Source: CAD feature listing. Evaluate the final solid. Frame: model axes, mm. A direction names the side the tool comes from. Round coordinates to 2 decimals unless told otherwise and drop trailing zeros. Write each loop counter-clockwise with the first axis right and the second up, starting at its lowest first coordinate (ties: lowest second). Pieces come first, ordered by that corner, then holes. Notation, with made-up numbers: M -40,22.25 L 2,22.25 A15 cw 2,49.25 Z; hole C -4.5,39 d4. An arc over 180 degrees is marked long. Use a Markdown table: item, result.
```python
from build123d import *

# Parameters (mm, degrees)
F0_W      = 4.724400118
F0_H      = 62.3315982521
F1_DEPTH  = 6.35
F2_R      = 2.53999
F4_DEPTH  = 1.27
F6_DEPTH  = 1.27
F8_DEPTH  = 25.4
F9_DEPTH  = 50.8
F11_DEPTH = 25.4
F13_DEPTH = 25.4
F15_DEPTH = 101.6


# Not quite as in the source:
# - a fillet or chamfer is up to 0.001 mm smaller than in the source, because OpenCascade refuses the exact size


with BuildPart() as f1:
    # F0 (on Top) → F1 (new body)
    with BuildSketch(Plane.XY):
        with Locations((2.362200059, 31.165799126)):
            Rectangle(F0_W, F0_H)
        with Locations((7.086600177, 31.165799126)):
            Rectangle(F0_W, F0_H)
        Polygon((4.724400118, 75.0454813242), (4.724400118, 62.3315982521), (9.448800236, 62.3315982521), align=None)
        Polygon((4.724400118, 75.0454813242), (0, 62.3315982521), (4.724400118, 62.3315982521), align=None)
        with BuildLine():
            Line((4.724400118, 0), (0, 0))
            Line((0, 0), (-20.32, 0))
            ThreePointArc((-20.32, 0), (-18.5239487758, -0.7439487758), (-17.78, -2.54))
            ThreePointArc((-17.78, -2.54), (-18.5239487758, -4.3360512242), (-20.32, -5.08))
            Line((-20.32, -5.08), (0, -5.08))
            Line((0, -5.08), (9.448800236, -5.08))
            Line((9.448800236, -5.08), (29.768800236, -5.08))
            ThreePointArc((29.768800236, -5.08), (27.228800236, -2.54), (29.768800236, 0))
            Line((29.768800236, 0), (9.448800236, 0))
            Line((9.448800236, 0), (4.724400118, 0))
        make_face()
        with BuildLine():
            Line((9.448800236, -5.08), (0, -5.08))
            Line((0, -5.08), (0, -43.18))
            ThreePointArc((0, -43.18), (4.724400118, -38.455599882), (9.448800236, -43.18))
            Line((9.448800236, -43.18), (9.448800236, -5.08))
        make_face()
        with BuildLine():
            ThreePointArc((-17.78, -2.54), (-18.5239487758, -0.7439487758), (-20.32, 0))
            Line((-20.32, 0), (-20.32, -5.08))
            ThreePointArc((-20.32, -5.08), (-18.5239487758, -4.3360512242), (-17.78, -2.54))
        make_face()
        with BuildLine():
            Line((-20.32, -5.08), (-20.32, 0))
            ThreePointArc((-20.32, 0), (-22.86, -2.54), (-20.32, -5.08))
        make_face()
        with BuildLine():
            Line((29.768800236, -5.08), (29.768800236, 0))
            ThreePointArc((29.768800236, 0), (27.228800236, -2.54), (29.768800236, -5.08))
        make_face()
        with BuildLine():
            ThreePointArc((32.308800236, -2.54), (31.5648514602, -0.7439487758), (29.768800236, 0))
            Line((29.768800236, 0), (29.768800236, -5.08))
            ThreePointArc((29.768800236, -5.08), (31.5648514602, -4.3360512242), (32.308800236, -2.54))
        make_face()
        with BuildLine():
            Line((9.448800236, -43.18), (0, -43.18))
            ThreePointArc((0, -43.18), (4.724400118, -47.904400118), (9.448800236, -43.18))
        make_face()
        with BuildLine():
            ThreePointArc((9.448800236, -43.18), (4.724400118, -38.455599882), (0, -43.18))
            Line((0, -43.18), (9.448800236, -43.18))
        make_face()
    extrude(amount=F1_DEPTH)

    # F2 (radius 2.54 in the source; OpenCascade refuses exactly that, so slightly less here)
    f2_edges = [f1.edges().sort_by_distance(p)[0] for p in [
        (0, -24.13, 6.35),
        (9.4488, -24.13, 6.35),
        (0, -24.13, 0),
        (9.4488, -24.13, 0),
        (19.6088, -5.08, 0),
        (19.6088, 0, 0),
        (-10.16, 0, 0),
        (19.6088, -5.08, 6.35),
        (19.6088, 0, 6.35),
        (-10.16, -5.08, 6.35),
        (-10.16, 0, 6.35),
        (-10.16, -5.08, 0),
    ]]
    fillet(f2_edges, radius=F2_R)

    # F3 (on face) → F4 (cut)
    with BuildSketch(Plane.XY.offset(6.35)):
        Polygon((0, 62.3315982521), (0, 0), (9.448800236, 0), (9.448800236, 62.3315982521), (4.724400118, 75.0454813242), align=None)
    extrude(amount=-F4_DEPTH, mode=Mode.SUBTRACT)

    # F5 (on face) → F6 (cut)
    with BuildSketch(Plane(origin=(0, 0, 0), x_dir=(1, 0, 0), z_dir=(0, 0, -1))):
        Polygon((9.448800236, 0), (0, 0), (0, -62.3315982521), (4.724400118, -75.0454813242), (9.448800236, -62.3315982521), align=None)
    extrude(amount=-F6_DEPTH, mode=Mode.SUBTRACT)

    # F7 (on face) → F8 (cut)
    with BuildSketch(Plane.XY.offset(5.08)):
        Polygon((4.724400118, 75.0454813242), (0, 62.3315982521), (9.448800236, 62.3315982521), align=None)
    extrude(amount=-F8_DEPTH, mode=Mode.SUBTRACT)

    # F9 (add): a face of the model
    f9_faces = [f1.faces().sort_by_distance(p)[0] for p in [
        (4.724400118, 62.3315982521, 3.175),
    ]]
    extrude(f9_faces, amount=F9_DEPTH)

    # F10 (on face) → F11 (cut)
    with BuildSketch(Plane.XY.offset(5.08)):
        Polygon((0, 102.5230064988), (4.724400118, 113.1315982521), (0, 113.1315982521), align=None)
        Polygon((9.448800236, 113.1315982521), (4.724400118, 113.1315982521), (9.448800236, 102.5230064988), align=None)
    extrude(amount=-F11_DEPTH, mode=Mode.SUBTRACT)

    # F12 (on face) → F13 (cut)
    with BuildSketch(Plane.XY.offset(5.08)):
        Polygon((4.724400118, 113.1315982521), (0, 102.5230064988), (9.448800236, 102.5230064988), align=None)
    extrude(amount=-F13_DEPTH, mode=Mode.SUBTRACT)

    # F14 (on face) → F15 (cut)
    with BuildSketch(Plane(origin=(0, 102.5230064988, 0), x_dir=(-1, 0, 0), z_dir=(0, 1, 0))):
        Polygon((0, 5.08), (-4.724400118, 5.08), (0, 3.175), align=None)
        Polygon((0, 1.27), (0, 3.175), (-4.724400118, 1.27), align=None)
        Polygon((-4.724400118, 1.27), (-9.448800236, 3.175), (-9.448800236, 1.27), align=None)
        Polygon((-9.448800236, 3.175), (-4.724400118, 5.08), (-9.448800236, 5.08), align=None)
    extrude(amount=-F15_DEPTH, mode=Mode.SUBTRACT)


solid = f1.part
```
Q1. Reachability of faces 1 (the cylindrical face through (8.72, -22.58, 5.59)), 2 (the flat face through (2.395, 52.434, 4.141)), 3 (the cylindrical face through (18.499, -4.356, 0.764)), 4 (the flat face through (0, 0.3, 3.2)), 5 (the cylindrical face through (-8.73, -4.356, 5.586)) from +Z, -Z, +X, -X, +Y, -Y: full face, straight path, thin tool, end or side. Return the list, or none.
Results are:
| item | result |
|---|---|
| face 1 | +Z, +X, -Y |
| face 2 | +Z, -X, +Y |
| face 3 | -Z, +X, -Y |
| face 4 | -X, +Y |
| face 5 | +Z, -X, -Y |
Q2. Line query: L1, parallel to Y at x = -9, z = 2.25; L2, parallel to Y at x = -6, z = 6; L3, parallel to X at y = -36, z = 5.25. Output: solid intervals per line, ascending.
Results are:
| item | result |
|---|---|
| L1 | -5.06 to -0.02 |
| L2 | -3.83 to -1.25 |
| L3 | 0.45 to 9 |
Q3. Section A-A on y = -36.5. Return loops of the section in (x, z), plus the area to 3 significant figures.
Results are:
| item | result |
|---|---|
| outline | M 0,2.54 A2.54 ccw 2.54,0 L 6.91,0 A2.54 ccw 9.45,2.54 L 9.45,3.81 A2.54 ccw 6.91,6.35 L 2.54,6.35 A2.54 ccw 0,3.81 Z |
| area | 54.5 mm^2 |
Q4. Section C-C on y = 43.5. Return loops of the section in (x, z) (3 decimals), plus the area to 3 significant figures.
Results are:
| item | result |
|---|---|
| outline | M 0,3.175 L 4.724,1.27 L 9.449,3.175 L 4.724,5.08 Z |
| area | 18.0 mm^2 |
Q5. First-contact query: pin 1 Ø0.6 at (x, z) = (15, 3.5) entering from -Y; pin 2 Ø0.7 at (x, y) = (4, 0.5) entering from -Z; pin 3 Ø1.5 at (x, z) = (-1, 1.5) entering from +Y. Flat tips, straight axial feed; report the tip coordinate or a pass-through.
Results are:
| item | result |
|---|---|
| pin 1 | y = -5.08 |
| pin 2 | z = 1.27 |
| pin 3 | y = -0.02 |
